```python
from build123d import *

# Parameters (mm, degrees)
SKETCH_W        = 97.65
SKETCH_H        = 74.5
PAD_DEPTH       = 6
SKETCH001_W     = 93.65
SKETCH001_H     = 70.5
POCKET_DEPTH    = 4
SKETCH002_R     = 4
PAD001_DEPTH    = 2.3
SKETCH003_R     = 1.85
POCKET001_DEPTH = 4.301
CHAMFER_SIZE    = 1.5
FILLET_R        = 2


with BuildPart() as part:
    # Sketch → Pad (new body)
    with BuildSketch(Plane.XY):
        Rectangle(SKETCH_W, SKETCH_H)
    extrude(amount=PAD_DEPTH)

    # Sketch001 → Pocket (cut)
    with BuildSketch(Plane.XY.offset(6)):
        Rectangle(SKETCH001_W, SKETCH001_H)
    extrude(amount=-POCKET_DEPTH, mode=Mode.SUBTRACT)

    # Sketch002 → Pad001 (new body)
    with BuildSketch(Plane.XY.offset(2)):
        with Locations((-40.375, 25.8)):
            Circle(SKETCH002_R)
        with Locations((40.375, 25.8)):
            Circle(SKETCH002_R)
        with Locations((40.375, -28.8)):
            Circle(SKETCH002_R)
        with Locations((-40.375, -28.8)):
            Circle(SKETCH002_R)
    extrude(amount=PAD001_DEPTH)

    # Sketch003 → Pocket001 (cut, through all)
    with BuildSketch(Plane.XY.offset(4.3)):
        with Locations((-40.375, 25.8)):
            Circle(SKETCH003_R)
        with Locations((40.375, -28.8)):
            Circle(SKETCH003_R)
        with Locations((40.375, 25.8)):
            Circle(SKETCH003_R)
        with Locations((-40.375, -28.8)):
            Circle(SKETCH003_R)
    extrude(amount=-POCKET001_DEPTH, mode=Mode.SUBTRACT)

    # Chamfer
    chamfer_edges = [part.edges().sort_by_distance(p)[0] for p in [
        (38.525, 25.8, 0),
        (-42.225, -28.8, 0),
        (38.525, -28.8, 0),
        (-42.225, 25.8, 0),
    ]]
    chamfer(chamfer_edges, length=CHAMFER_SIZE)

    # Fillet
    fillet_edges = [part.edges().sort_by_distance(p)[0] for p in [
        (48.825, 0, 0),
        (48.825, -37.25, 3),
        (0, -37.25, 0),
        (0, 37.25, 0),
        (-48.825, 0, 0),
        (-48.825, 37.25, 3),
        (-48.825, -37.25, 3),
        (48.825, 37.25, 3),
    ]]
    fillet(fillet_edges, radius=FILLET_R)


solid = part.part
```
Geometry check sheet. Reference: the model listing, model coordinates, mm. A direction names the side the tool comes from. Round coordinates to 2 decimals unless told otherwise and drop trailing zeros. Order: outer loops, then holes, each group sorted by start corner. A loop starts at its lowest first (then second) coordinate and runs counter-clockwise, first axis right, second up. Notation, with made-up numbers: (85.5, -12) - (112.5, -12) arc R24 ccw to (112.5, 21) - close; hole circle Ø8 at (-36, 10.5). An arc over 180 degrees is marked (long way). Use a Markdown table: item, result. Add a question column.
(1) Sectioned sample at A-A, the plane z = 3. Count the separate pieces of the cut face and the enclosed holes in it, and give its area (3 significant figures).
(2) Release check for a two-part mould opening along Y. For faces 3 (the flat face through (46.825, 0, 4)), 4 (the flat face through (48.825, 0, 4)), 5 (the cylindrical face through (48.2, 36.7, 4)) record: pulls with the +Y half, pulls with the -Y half, needs draft (parallel to the pull), parting line crosses it, or undercut.
(3) Sectioned sample at C-C, the plane x = -12. Enter the section's corners in (y, z).
(4) Tool access check on faces 1 (the flat face through (-48.825, 0, 4)), 2 (the cylindrical face through (37.2, 23.37, 3.13)). Record the directions out of +Z, -Z, +X, -X, +Y, -Y that give a thin tool (end or side, any length) a straight path to the whole face; none if there is none.
(5) Material ranges on line 1 along Y through (x, z) = (23, 4.95); line 2 along X through (y, z) = (-24, 4.05) (3 decimals); line 3 along Z through (x, y) = (-43, 15), recorded low to high. Write a range as [from, to].
(6) Depth check by flat-ended pin: pin 1 (3 mm diameter, centred on x = 40.375, y = 25.8, fed in from -Z); pin 2 (5 mm diameter, centred on x = -40.375, y = 25.8, fed in from -Z); pin 3 (9 mm diameter, centred on x = 39.5, y = -27.5, fed in from +Z); pin 4 (1 mm diameter, centred on x = 17, y = -24.5, fed in from +Z). Enter the tip coordinate at first touch or a pass-through.
(7) Sectioned sample at D-D, the plane y = -5. Enter the section's corners in (x, z) (3 decimals), and give its area (3 significant figures).
Answers below:
| question | item | result |
|---|---|---|
| 1 | separate pieces | 5 |
| 1 | enclosed holes | 5 |
| 1 | area | 827 mm² |
| 2 | face 3 | undercut |
| 2 | face 4 | needs draft |
| 2 | face 5 | pulls with the +Y half |
| 3 | outline | (-37.25, 2) arc R2 ccw to (-35.25, 0) - (35.25, 0) arc R2 ccw to (37.25, 2) - (37.25, 6) - (35.25, 6) - (35.25, 2) - (-35.25, 2) - (-35.25, 6) - (-37.25, 6) - close |
| 4 | face 1 | +Z, -Z, -X, +Y, -Y |
| 4 | face 2 | +Z |
| 5 | line 1 | [-37.25, -35.25], [35.25, 37.25] |
| 5 | line 2 | [-48.825, -46.825], [46.825, 48.825] |
| 5 | line 3 | [0, 2] |
| 6 | pin 1 | through |
| 6 | pin 2 | z = 0.85 |
| 6 | pin 3 | z = 4.3 |
| 6 | pin 4 | z = 2 |
| 7 | outline | (-48.825, 2) arc R2 ccw to (-46.825, 0) - (46.825, 0) arc R2 ccw to (48.825, 2) - (48.825, 6) - (46.825, 6) - (46.825, 2) - (-46.825, 2) - (-46.825, 6) - (-48.825, 6) - close |
| 7 | area | 210 mm² |
